The figure shows three views and two pictorial views of one solid part (mm, origin at its lowest corner). Answer the questions. Round coordinates to 2 decimals unless told otherwise and drop trailing zeros. Write each loop counter-clockwise with the first axis right and the second up, starting at its lowest first coordinate (ties: lowest second). Pieces come first, ordered by that corner, then holes.
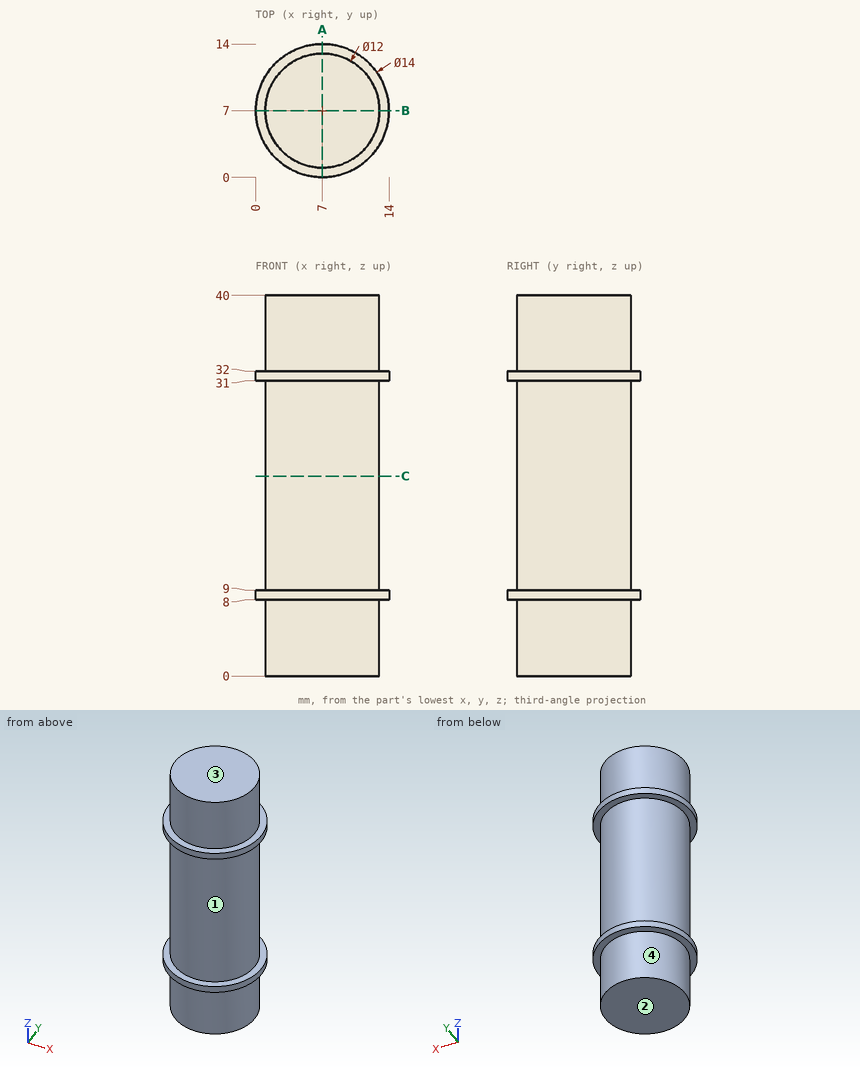
Q1. Determine the mould class of the marked faces 1, 2, 3 and 4 for opening direction Z: pulls with the +Z half, pulls with the -Z half, needs draft (parallel to the pull), parting line crosses it, or undercut.
Verdict:
face 1: undercut
face 2: pulls with the -Z half
face 3: pulls with the +Z half
face 4: needs draft
Q2. Straight lines are drawn through the part: probe 1 along Z at (x, y) = (1, 5); probe 2 along X at (y, z) = (7.25, 25.5); probe 3 along Y at (x, z) = (7.75, 17). For each, find the intervals that lie inside material, in ascending order.
Verdict:
probe 1: z = 8 to 9, 31 to 32
probe 2: x = 1.01 to 12.99
probe 3: y = 1.05 to 12.95
Q3. Section C-C (z = 21) is taken. Determine the outline of the cut face in (x, y), then the cut area to 3 significant figures.
Verdict:
outline: circle Ø12 at (7, 7)
area: 113 mm2
Q4. Section A-A (x = 7) is taken. Determine the outline of the cut face in (y, z).
Verdict:
outline: (0, 8) - (1, 8) - (1, 0) - (13, 0) - (13, 8) - (14, 8) - (14, 9) - (13, 9) - (13, 31) - (14, 31) - (14, 32) - (13, 32) - (13, 40) - (1, 40) - (1, 32) - (0, 32) - (0, 31) - (1, 31) - (1, 9) - (0, 9) - close
Q5. Flat-ended cylindrical pins translate along their axes: pin 1 Ø1 at (y, z) = (9, 28) entering from +X; pin 2 Ø5 at (x, z) = (9, 21) entering from -Y; pin 3 Ø2 at (x, z) = (12.5, 16.5) entering from +Y. Find the tip coordinate at first contact, or state that the pin passes through.
Verdict:
pin 1: stops at x = 12.81
pin 2: stops at y = 1
pin 3: stops at y = 10.97
